from build123d import *

# Parameters (mm, degrees)
CYLINDER030_R     = 1.6
CYLINDER030_DEPTH = 28
BOX040_W          = 8
BOX040_H          = 10.5
BOX040_DEPTH      = 2.5
CYLINDER007_R     = 1.1
CYLINDER007_DEPTH = 28
CYLINDER006_R     = 1.1
CYLINDER006_DEPTH = 28
CYLINDER005_R     = 1.6
CYLINDER005_DEPTH = 28
CYLINDER004_R     = 3
CYLINDER004_DEPTH = 4
BOX009_W          = 4
BOX009_H          = 52
BOX009_DEPTH      = 1.5
BOX008_W          = 77
BOX008_H          = 48
BOX008_DEPTH      = 40
FILLET002_R       = 8
BOX005_W          = 8
BOX005_H          = 52
BOX005_DEPTH      = 26
FILLET003_R       = 9


with BuildPart() as cylinder030:
    # Cylinder030 → Cylinder030 (new body)
    with BuildSketch(Plane(origin=(74, 76, -28), x_dir=(1, 0, 0), z_dir=(0, 0, 1))):
        Circle(CYLINDER030_R)
    extrude(amount=CYLINDER030_DEPTH)


with BuildPart() as cut030:
    # Box040 → Box040 (new body)
    with BuildSketch(Plane(origin=(70, 71.5, -26), x_dir=(1, 0, 0), z_dir=(0, 0, 1))):
        with Locations((4, 5.25)):
            Rectangle(BOX040_W, BOX040_H)
    extrude(amount=BOX040_DEPTH)

    # Cut030: cut Cylinder030
    add(cylinder030.part, mode=Mode.SUBTRACT)


with BuildPart() as cut030_1:
    # Cut030 placement: moved
    add(cut030.part.moved(Location((0, 0, 26))))


with BuildPart() as cylinder007:
    # Cylinder007 → Cylinder007 (new body)
    with BuildSketch(Plane(origin=(74, 118, -26), x_dir=(1, 0, 0), z_dir=(0, 0, 1))):
        Circle(CYLINDER007_R)
    extrude(amount=CYLINDER007_DEPTH)


with BuildPart() as fusion007:
    # Cylinder006 → Cylinder006 (new body)
    with BuildSketch(Plane(origin=(74, 94, -26), x_dir=(1, 0, 0), z_dir=(0, 0, 1))):
        Circle(CYLINDER006_R)
    extrude(amount=CYLINDER006_DEPTH)

    # Fusion007: union Cylinder007
    add(cylinder007.part)


with BuildPart() as cylinder005:
    # Cylinder005 → Cylinder005 (new body)
    with BuildSketch(Plane(origin=(74, 79, -26), x_dir=(1, 0, 0), z_dir=(0, 0, 1))):
        Circle(CYLINDER005_R)
    extrude(amount=CYLINDER005_DEPTH)


with BuildPart() as fusion006:
    # Cylinder004 → Cylinder004 (new body)
    with BuildSketch(Plane(origin=(74, 79, -26), x_dir=(1, 0, 0), z_dir=(0, 0, 1))):
        Circle(CYLINDER004_R)
    extrude(amount=CYLINDER004_DEPTH)

    # Fusion006: union Cylinder005
    add(cylinder005.part)


with BuildPart() as fusion006_1:
    # Fusion006 placement: moved
    add(fusion006.part.moved(Location((0, -3, 0))))


with BuildPart() as box009:
    # Box009 → Box009 (new body)
    with BuildSketch(Plane(origin=(72, 71.5, -26), x_dir=(1, 0, 0), z_dir=(0, 0, 1))):
        with Locations((2, 26)):
            Rectangle(BOX009_W, BOX009_H)
    extrude(amount=BOX009_DEPTH)


with BuildPart() as fillet002:
    # Box008 → Box008 (new body)
    with BuildSketch(Plane(origin=(62, 82, -27), x_dir=(1, 0, 0), z_dir=(0, 0, 1))):
        with Locations((38.5, 24)):
            Rectangle(BOX008_W, BOX008_H)
    extrude(amount=BOX008_DEPTH)

    # Fillet002
    fillet002_edges = [fillet002.edges().sort_by_distance(p)[0] for p in [
        (100.5, 82, -27),
        (100.5, 82, 13),
        (100.5, 130, -27),
        (100.5, 130, 13),
    ]]
    fillet(fillet002_edges, radius=FILLET002_R)


with BuildPart() as fillet002_1:
    # Fillet002 placement: moved
    add(fillet002.part.moved(Location((0, 0, 4))))


with BuildPart() as fusion034:
    # Box005 → Box005 (new body)
    with BuildSketch(Plane(origin=(70, 71.5, -26), x_dir=(1, 0, 0), z_dir=(0, 0, 1))):
        with Locations((4, 26)):
            Rectangle(BOX005_W, BOX005_H)
    extrude(amount=BOX005_DEPTH)

    # Cut002: cut Fillet002
    add(fillet002_1.part, mode=Mode.SUBTRACT)

    # Fillet003
    fillet003_edges = [fusion034.edges().sort_by_distance(p)[0] for p in [
        (74, 71.5, -26),
    ]]
    fillet(fillet003_edges, radius=FILLET003_R)

    # Cut003: cut Box009
    add(box009.part, mode=Mode.SUBTRACT)

    # Cut007: cut Fusion006
    add(fusion006_1.part, mode=Mode.SUBTRACT)

    # Cut008: cut Fusion007
    add(fusion007.part, mode=Mode.SUBTRACT)

    # Fusion034: union Cut030
    add(cut030_1.part)


solid = fusion034.part
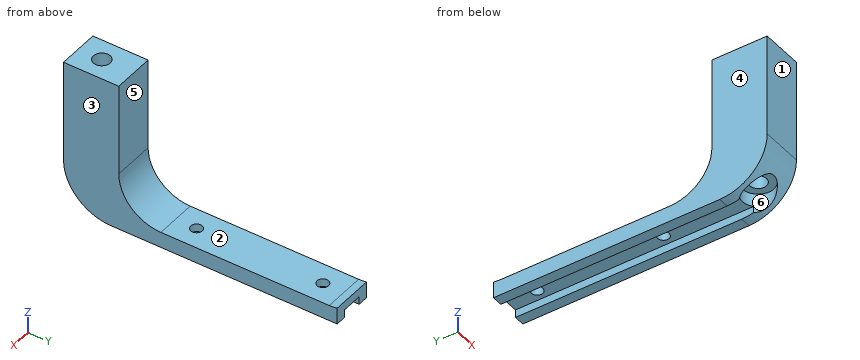
Input: part model. Units: mm. Frame: model coordinates. Face numbers are marked on the shaded views. A direction names the side the tool comes from. Give positions to 0.01 mm unless a question says otherwise; leave off trailing zeros. Write each loop counter-clockwise with the first axis right and the second up, starting at its lowest first coordinate (ties: lowest second). Pieces come first, ordered by that corner, then holes. Notation, with made-up numbers: (47, 35) -> (62, 35) arc R30 ccw to (62, 71) -> close; hole circle Ø1 at (57.5, 77). An arc over 180 degrees is marked (long way). Use one line per item in the form item = value. Start each with the question number.
1) Section query D-D on y = 76. Return the cut outline in (x, z).
2) Ray query, probe 1 along Y at (x, z) = (74, -23.3); probe 2 along Z at (x, y) = (71, 95.5); probe 3 along X at (y, z) = (118, -24). Return the intervals inside material, ascending. Write a range as from..to.
3) Pin query (flat end, axial travel): pin 1 (2.5 mm diameter, centred on x = 73, z = -6.5, fed in from +Y); pin 2 (2.5 mm diameter, centred on x = 74.5, y = 109, fed in from +Z). Return the tip coordinate at first contact, or that it passes through.
4) Section query C-C on y = 102. Return the cut outline in (x, z), then the cut area to 3 significant figures.
5) Section query B-B on z = -5.5. Return the cut outline in (x, y).
6) Section query A-A on y = 94. Return the cut outline in (x, z).
7) Draft query along Y for the marked faces 1, 2 and 3. Return one class per face: pulls with the +Y half, pulls with the -Y half, needs draft (parallel to the pull), parting line crosses it, or undercut.
8) Set-up query: the marked faces 4, 5 and 6. Return all of +Z, -Z, +X, -X, +Y, -Y with unobstructed straight access to the full face (end or side cutting, diameter ignored); none if empty.
Outcome:
q1.outline = (70, -24.79) -> (71, -24.79) -> (71, -22) -> (72.4, -22) -> (72.4, 2.5) -> (70, 2.5) -> close; (75.6, -22) -> (77, -22) -> (77, -24.79) -> (78, -24.79) -> (78, 2.5) -> (75.6, 2.5) -> close
q2.probe_1 = 79..92.9, 95.1..116.9, 119.1..123.5
q2.probe_2 = -26..-23
q2.probe_3 = 70..72.9, 75.1..78
q3.pin_1 = 82
q3.pin_2 = -23
q4.outline = (70, -26) -> (72, -26) -> (72, -24.5) -> (76, -24.5) -> (76, -26) -> (78, -26) -> (78, -23) -> (70, -23) -> close
q4.area = 18.0 mm^2
q5.outline = (70, 71.5) -> (78, 71.5) -> (78, 82) -> (70, 82) -> close; hole circle Ø3.2 at (74, 76)
q6.outline = (70, -26) -> (72, -26) -> (72, -24.5) -> (72.9, -24.5) -> (72.9, -23) -> (70, -23) -> close; (75.1, -24.5) -> (76, -24.5) -> (76, -26) -> (78, -26) -> (78, -23) -> (75.1, -23) -> close
q7.face_1 = pulls with the -Y half
q7.face_2 = undercut
q7.face_3 = needs draft
q8.face_4 = +Z, -Z, -X, +Y, -Y
q8.face_5 = +Z, +X, -X, +Y
q8.face_6 = -Z
